```python
from build123d import *

# Parameters (mm, degrees)
PAD_DEPTH       = 9
SKETCH001_W     = 40
SKETCH001_H     = 40
PAD001_DEPTH    = 3
SKETCH002_W     = 56.425
SKETCH002_H     = 47
PAD002_DEPTH    = 3
SKETCH003_W     = 34.2
SKETCH003_H     = 30.9
POCKET_DEPTH    = 5
POCKET001_DEPTH = 5


with BuildPart() as part:
    # Sketch → Pad (new body)
    with BuildSketch(Plane.XZ):
        Polygon((-20, 0), (20, 0), (28.2125, 76.042319), (-28.2125, 76.042319), align=None)
    extrude(amount=PAD_DEPTH)

    # Sketch001 (on Face2 of Pad) → Pad001 (join)
    with BuildSketch(Plane(origin=(0, 0, 0), x_dir=(1, 0, 0), z_dir=(0, 0, -1))):
        with Locations((0, 20)):
            Rectangle(SKETCH001_W, SKETCH001_H)
    extrude(amount=-PAD001_DEPTH)

    # Sketch002 (on Face2 of Pad001) → Pad002 (join)
    with BuildSketch(Plane(origin=(0, 0, 76.042319), x_dir=(-1, 0, 0), z_dir=(0, 0, 1))):
        with Locations((0, 23.5)):
            Rectangle(SKETCH002_W, SKETCH002_H)
    extrude(amount=-PAD002_DEPTH)

    # Sketch003 (on Face14 of Pad002) → Pocket (cut)
    with BuildSketch(Plane(origin=(0, 0, 76.042319), x_dir=(-1, 0, 0), z_dir=(0, 0, 1))):
        with Locations((0, 26.55)):
            Rectangle(SKETCH003_W, SKETCH003_H)
    extrude(amount=-POCKET_DEPTH, mode=Mode.SUBTRACT)

    # Sketch004 (on Face5 of Pocket) → Pocket001 (cut)
    with BuildSketch(Plane(origin=(0, 0, 0), x_dir=(1, 0, 0), z_dir=(0, 0, -1))):
        Polygon((-16, 12), (16, 12), (10, 37), (-10, 37), align=None)
    extrude(amount=-POCKET001_DEPTH, mode=Mode.SUBTRACT)


solid = part.part
```
Geometry check sheet. Reference: the model listing, model coordinates, mm. A direction names the side the tool comes from. Give positions to 0.01 mm unless a question says otherwise; leave off trailing zeros. Order: outer loops, then holes, each group sorted by start corner. A loop starts at its lowest first (then second) coordinate and runs counter-clockwise, first axis right, second up.
1. Section check B-B, the plane y = -39. Enter the section's corners in (x, z).
2. Thickness scan on L1, parallel to Y at x = -25.5, z = 72; L2, parallel to Z at x = 22, y = -34; L3, parallel to Z at x = -13.5, y = -35. Record the ranges inside material, lowest first.
3. Release check for a two-part mould opening along X. For faces 1 (the face through (0, -40, 1)), 2 (the face through (0, -12, 1)), 3 (the face through (-24, -4.44, 37.03)) record: pulls with the +X half, pulls with the -X half, needs draft (parallel to the pull), parting line crosses it, or undercut.
4. Access from +Z, -Z, +X, -X, +Y, -Y to the whole of each face (thin tool, end or side, straight path). Record for faces 4 (the face through (0, -11.1, 75)), 5 (the face through (20, -24, 1)), 6 (the face through (-12.96, -24.67, 1.48)), 7 (the face through (0, -38, 3)), 8 (the face through (-20, -24, 1)).
5. Section check C-C, the plane y = -25.5. Enter the section's corners in (x, z).
6. Gauge pin test, flat ends, axial feed: pin 1 Ø6 at (x, z) = (16, 62) entering from -Y; pin 2 Ø14 at (x, y) = (-7, -30.5) entering from -Z; pin 3 Ø1.5 at (x, z) = (5.5, 1.5) entering from -Y; pin 4 Ø2.5 at (y, z) = (-29, 1) entering from -X. Record the tip position at first contact, or that the pin passes through.
7. Section check D-D, the plane x = -14.5. Enter the section's corners in (y, z).
8. Section check A-A, the plane x = -1.5. Enter the section's corners in (y, z), and give its area (3 significant figures).
Values follow:
1. outline: (-28.21, 73.04) - (-17.1, 73.04) - (-17.1, 76.04) - (-28.21, 76.04) - close; (-20, 0) - (20, 0) - (20, 3) - (-20, 3) - close; (17.1, 73.04) - (28.21, 73.04) - (28.21, 76.04) - (17.1, 76.04) - close
2. L1: y = -9 to 0
2. L2: z = 73.04 to 76.04
2. L3: z = 0 to 3
3. face 1: needs draft
3. face 2: undercut
3. face 3: pulls with the -X half
4. face 4: +Z
4. face 5: -Z, +X, -Y
4. face 6: +Z, -Z
4. face 7: +X, -X, -Y
4. face 8: -Z, -X, -Y
5. outline: (-28.21, 73.04) - (-17.1, 73.04) - (-17.1, 76.04) - (-28.21, 76.04) - close; (-20, 0) - (-12.76, 0) - (-12.76, 3) - (-20, 3) - close; (12.76, 0) - (20, 0) - (20, 3) - (12.76, 3) - close; (17.1, 73.04) - (28.21, 73.04) - (28.21, 76.04) - (17.1, 76.04) - close
6. pin 1: stops at y = -9
6. pin 2: stops at z = 0
6. pin 3: stops at y = -40
6. pin 4: stops at x = -20
7. outline: (-47, 73.04) - (-42, 73.04) - (-42, 76.04) - (-47, 76.04) - close; (-40, 0) - (-18.25, 0) - (-18.25, 3) - (-40, 3) - close; (-12, 0) - (0, 0) - (0, 76.04) - (-11.1, 76.04) - (-11.1, 73.04) - (-9, 73.04) - (-9, 3) - (-12, 3) - close
8. outline: (-47, 73.04) - (-42, 73.04) - (-42, 76.04) - (-47, 76.04) - close; (-40, 0) - (-37, 0) - (-37, 3) - (-40, 3) - close; (-12, 0) - (0, 0) - (0, 76.04) - (-11.1, 76.04) - (-11.1, 73.04) - (-9, 73.04) - (-9, 3) - (-12, 3) - close
8. area: 724 mm2
